Can you work these out from the model? Positions are in its coordinate system, mm. A direction names the side the tool comes from. Give positions to 0.01 mm unless a question says otherwise; leave off trailing zeros. Write each loop counter-clockwise with the first axis right and the second up, starting at its lowest first coordinate (ties: lowest second). Pieces come first, ordered by that corner, then holes.
```python
from build123d import *

# Parameters (mm, degrees)
BOSS_EXTRUDE1_DEPTH = 9
SKETCH2_R           = 2.25
CUT_EXTRUDE1_DEPTH  = 16.5
SKETCH2_3_R         = 3.75
SKETCH2_3_R_2       = 2.25
CUT_EXTRUDE2_DEPTH  = 1
SKETCH3_R           = 3
BOSS_EXTRUDE2_DEPTH = 12


with BuildPart() as part:
    # Sketch1 → Boss-Extrude1 (new body)
    with BuildSketch(Plane.XY):
        Polygon((0, 0), (17.616685226, 9.5), (27.6, 9.5), (27.6, 14.5), (35.6, 14.5), (35.6, 16.5), (26.6, 16.5), (19.116685226, 11.5), (18.116685226, 11.5), (13.116685226, 17.5), (11.616685226, 17.5), (0, 0.25), align=None)
    extrude(amount=BOSS_EXTRUDE1_DEPTH)

    # Sketch2 → Cut-Extrude1 (cut)
    with BuildSketch(Plane(origin=(0, 16.5, 0), x_dir=(1, 0, 0), z_dir=(0, 1, 0))):
        with Locations(Location((31.6, -4.5, 0), (0, 0, 270))):
            Circle(SKETCH2_R)
        Polygon((0, 0), (0, -4), (8.616685226, 0), align=None)
        Polygon((0, -5), (8.616685226, -9), (0, -9), align=None)
    extrude(amount=-CUT_EXTRUDE1_DEPTH, mode=Mode.SUBTRACT)

    # Sketch2<3> → Cut-Extrude2 (cut)
    with BuildSketch(Plane(origin=(0, 16.5, 0), x_dir=(1, 0, 0), z_dir=(0, 1, 0))):
        with Locations(Location((31.6, -4.5, 0), (0, 0, 270))):
            Circle(SKETCH2_3_R)
        with Locations(Location((31.6, -4.5, 0), (0, 0, 270))):
            Circle(SKETCH2_3_R_2, mode=Mode.SUBTRACT)
    extrude(amount=-CUT_EXTRUDE2_DEPTH, mode=Mode.SUBTRACT)

    # Sketch3 → Boss-Extrude2 (add)
    with BuildSketch(Plane(origin=(16.347551937, 13.622959947, 0), x_dir=(0, 0, -1), z_dir=(0.768221279597376, 0.6401843996644799, 0))):
        with Locations(Location((-4.5, 1.046775136, 0), (0, 0, 270))):
            Circle(SKETCH3_R)
    extrude(amount=BOSS_EXTRUDE2_DEPTH)


solid = part.part
```
1) Suppose I cut it at D-D on y = 10. Write out the boundary of the cut face in (x, z), plus the area to 3 significant figures.
Values follow:
outline: (6.57, 0.95) - (8.62, 0) - (27.6, 0) - (27.6, 9) - (8.62, 9) - (6.57, 8.05) - close
area: 187 mm2
2) Suppose I cut it at C-C on z = 2.75. Write out the boundary of the cut face in (x, y), plus the area to 3 significant figures.
Values follow:
outline: (2.69, 1.45) - (17.62, 9.5) - (27.6, 9.5) - (27.6, 14.5) - (30.19, 14.5) - (30.19, 15.5) - (28.28, 15.5) - (28.28, 16.5) - (26.6, 16.5) - (19.12, 11.5) - (18.12, 11.5) - (17.24, 12.56) - (26.46, 20.24) - (23.34, 23.98) - (14.12, 16.3) - (13.12, 17.5) - (11.62, 17.5) - (2.69, 4.25) - close; (33.01, 14.5) - (35.6, 14.5) - (35.6, 16.5) - (34.92, 16.5) - (34.92, 15.5) - (33.01, 15.5) - close
area: 217 mm2
3) For pin 1 Ø3 at (x, y) = (23, 20.5) entering from +Z; pin 2 Ø4.5 at (x, z) = (33, 6.5) entering from +Y; pin 3 Ø4 at (y, z) = (6.5, 6) entering from -X, each with a flat end and sliding along its axis, tell me the tip position at first contact or that it passes through.
Values follow:
pin 1: stops at z = 7.5
pin 2: stops at y = 16.5
pin 3: stops at x = 2.86
4) Suppose I cut it at B-B on z = 4.5. Write out the boundary of the cut face in (x, y).
Values follow:
outline: (0, 0) - (17.62, 9.5) - (27.6, 9.5) - (27.6, 14.5) - (29.35, 14.5) - (29.35, 15.5) - (27.85, 15.5) - (27.85, 16.5) - (26.6, 16.5) - (19.12, 11.5) - (18.12, 11.5) - (17.6, 12.12) - (26.82, 19.8) - (22.98, 24.41) - (13.76, 16.73) - (13.12, 17.5) - (11.62, 17.5) - (0, 0.25) - close; (33.85, 14.5) - (35.6, 14.5) - (35.6, 16.5) - (35.35, 16.5) - (35.35, 15.5) - (33.85, 15.5) - close
5) Suppose I cut it at A-A on x = 31.6. Write out the boundary of the cut face in (y, z).
Values follow:
outline: (14.5, 0) - (16.5, 0) - (16.5, 0.75) - (15.5, 0.75) - (15.5, 2.25) - (14.5, 2.25) - close; (14.5, 6.75) - (15.5, 6.75) - (15.5, 8.25) - (16.5, 8.25) - (16.5, 9) - (14.5, 9) - close
6) For faces 1 (the face through (15.1, 15.12, 1.44)), 2 (the face through (18.6, 11.5, 4.4)), 3 (the face through (12, 17.5, 4)), 4 (the face through (27.6, 12, 4)), which set-ups out of +Z, -Z, +X, -X, +Y, -Y let a thin tool reach every point of the face, with its end or its side?
Values follow:
face 1: none
face 2: +Z, -Z
face 3: +Z, -Z, -X, +Y
face 4: +Z, -Z, +X, -Y
7) Please list where these lines run through material, in increasing order: L1, parallel to Y at x = 25, z = 2.5; L2, parallel to Y at x = 12.5, z = 3.5; L3, parallel to Z at x = 25.5, y = 19.25.
Values follow:
L1: y = 9.5 to 15.43, 19.29 to 21.98
L2: y = 6.74 to 17.5
L3: z = 2.97 to 6.03
8) If we mould it in two halves opening along X, with no side actions, what happens to faces 5 (the face through (5.6, 5.6, 7.6)), 6 (the face through (29, 15.5, 4)), 7 (the face through (16, 11, 0))? For each: +X half, -X half, draft (parallel to the pull), parting line (faces both ways), or undercut.
Values follow:
face 5: -X half
face 6: undercut
face 7: draft
